Work out the finished part from the listing and answer in its coordinate system (mm). A direction names the side the tool comes from. Give positions to 0.01 mm unless a question says otherwise; leave off trailing zeros. Order: outer loops, then holes, each group sorted by start corner. A loop starts at its lowest first (then second) coordinate and runs counter-clockwise, first axis right, second up. Notation, with made-up numbers: (-36.75, 73) - (19.25, 73) arc R6 ccw to (19.25, 78) - close; hole circle Ø8 at (40.25, 50). An arc over 180 degrees is marked (long way). Write each question's results on one line, items separated by ' | '.
from build123d import *

# Parameters (mm, degrees)
SKETCH1_R           = 5
SKETCH1_R_2         = 2.5
BOSS_EXTRUDE2_DEPTH = 15
SKETCH2_W           = 6
SKETCH2_H           = 38.915837439
CUT_EXTRUDE1_DEPTH  = 11
CUT_EXTRUDE2_START  = -4.5
SKETCH3_R           = 4.6
SKETCH3_R_2         = 2.5
CUT_EXTRUDE2_DEPTH  = 6
CUT_EXTRUDE3_START  = -10.5
SKETCH4_R           = 4.6
SKETCH4_R_2         = 2.5
CUT_EXTRUDE3_DEPTH  = 6
BOSS_EXTRUDE3_DEPTH = 21
CUT_EXTRUDE4_DEPTH  = 67.015153021
BOSS_EXTRUDE4_START = -15.5
SKETCH8_R           = 6
BOSS_EXTRUDE4_DEPTH = 5.5


with BuildPart() as part:
    # Sketch1 → Boss-Extrude2 (new body)
    with BuildSketch(Plane(origin=(0, 0, 0), x_dir=(0, 0, -1), z_dir=(1, 0, 0))):
        with BuildLine():
            Line((0, -7), (4.514898748, -15.922762425))
            ThreePointArc((4.514898748, -15.922762425), (1.88507796, -23.910457261), (9.571950369, -20.5))
            Line((9.571950369, -20.5), (30.826440892, -20.5))
            ThreePointArc((30.826440892, -20.5), (36.979627599, -21.988417026), (38.792064121, -15.922762425))
            Line((38.792064121, -15.922762425), (38.792064121, 29.077237575))
            Line((38.792064121, 29.077237575), (17.792064121, 29.077237575))
            Line((17.792064121, 29.077237575), (17.792064121, 7))
            Line((17.792064121, 7), (0, 7))
            ThreePointArc((0, 7), (-7, 0), (0, -7))
        make_face()
        Circle(SKETCH1_R, mode=Mode.SUBTRACT)
        with Locations((4.971950369, -20.5)):
            Circle(SKETCH1_R_2, mode=Mode.SUBTRACT)
        with Locations((34.687787808, -18)):
            Circle(SKETCH1_R_2, mode=Mode.SUBTRACT)
    extrude(amount=BOSS_EXTRUDE2_DEPTH)

    # Sketch2 → Cut-Extrude1 (cut)
    with BuildSketch(Plane.XZ.offset(20.5)):
        with Locations((7.5, -19.829869089)):
            Rectangle(SKETCH2_W, SKETCH2_H)
    extrude(amount=-CUT_EXTRUDE1_DEPTH, mode=Mode.SUBTRACT)

    # Sketch3 → Cut-Extrude2 (cut)
    with BuildSketch(Plane.ZY.offset(CUT_EXTRUDE2_START)):
        with Locations((-4.971950369, -20.5)):
            Circle(SKETCH3_R)
        with Locations(Location((-4.971950369, -20.5, 0), (0, 0, 180))):
            Circle(SKETCH3_R_2, mode=Mode.SUBTRACT)
    extrude(amount=-CUT_EXTRUDE2_DEPTH, mode=Mode.SUBTRACT)

    # Sketch4 → Cut-Extrude3 (cut)
    with BuildSketch(Plane(origin=(15, 0, 0), x_dir=(0, 0, -1), z_dir=(1, 0, 0)).offset(CUT_EXTRUDE3_START)):
        with Locations((34.687787808, -18)):
            Circle(SKETCH4_R)
        with Locations((34.687787808, -18)):
            Circle(SKETCH4_R_2, mode=Mode.SUBTRACT)
    extrude(amount=CUT_EXTRUDE3_DEPTH, mode=Mode.SUBTRACT)

    # Sketch6 → Boss-Extrude3 (add)
    with BuildSketch(Plane(origin=(0, 0, -38.792064121), x_dir=(-1, 0, 0), z_dir=(0, 0, -1))):
        with BuildLine():
            ThreePointArc((0, 29.077237575), (-7.5, 44.40818947), (-15, 29.077237575))
            Line((-15, 29.077237575), (-8.914213562, 29.077237575))
            ThreePointArc((-8.914213562, 29.077237575), (-11.20909144, 39.624399885), (-1.5, 34.90818947))
            ThreePointArc((-1.5, 34.90818947), (-2.783789584, 31.199098029), (-6.085786438, 29.077237575))
            Line((-6.085786438, 29.077237575), (0, 29.077237575))
        make_face()
    extrude(amount=-BOSS_EXTRUDE3_DEPTH)

    # Sketch7 → Cut-Extrude4 (cut, through all)
    with BuildSketch(Plane(origin=(0, 0, -38.792064121), x_dir=(-1, 0, 0), z_dir=(0, 0, -1))):
        with BuildLine():
            Line((-8.914213562, 29.077237575), (-6.085786438, 29.077237575))
            ThreePointArc((-6.085786438, 29.077237575), (-7.5, 28.90818947), (-8.914213562, 29.077237575))
        make_face()
    extrude(amount=-CUT_EXTRUDE4_DEPTH, mode=Mode.SUBTRACT)

    # Sketch8 → Boss-Extrude4 (add)
    with BuildSketch(Plane(origin=(0, 0, -38.792064121), x_dir=(-1, 0, 0), z_dir=(0, 0, -1)).offset(BOSS_EXTRUDE4_START)):
        with Locations((-7.5, 34.90818947)):
            Circle(SKETCH8_R)
    extrude(amount=-BOSS_EXTRUDE4_DEPTH)


solid = part.part
1. A cutting plane is placed at A-A, the plane y = 0. Write down the section's boundary in (x, z).
Answer list:
outline: (0, -38.79) - (15, -38.79) - (15, -5) - (0, -5) - close; (0, 5) - (15, 5) - (15, 7) - (0, 7) - close
2. A cutting plane is placed at C-C, the plane z = -27. Write down the section's boundary in (x, y), then the cut area to 3 significant figures.
Answer list:
outline: (0, -20.5) - (4.5, -20.5) - (4.5, -9.5) - (10.5, -9.5) - (10.5, -20.5) - (15, -20.5) - (15, 29.08) arc R9.5 ccw (long way) to (0, 29.08) - close; hole circle Ø12 at (7.5, 34.91) | area: 810 mm^2
3. Given P1, Ø4, axis at x = 1, z = -6.5, coming from the +Y side; P2, Ø2, axis at x = 0, z = -34.5, coming from the +Y side; P3, Ø5, axis at y = 22, z = -27, coming from the -X side; P4, Ø6, axis at y = 0, z = 0, coming from the +X side, each flat-ended and moving along its own axis, determine where each tip first touches the part or whether it passes through.
Answer list:
P1: y = 7 | P2: y = 41.84 | P3: x = 0 | P4: through
4. A cutting plane is placed at B-B, the plane z = -36. Write down the section's boundary in (x, y), then the cut area to 3 significant figures.
Answer list:
outline: (0, -22.41) - (4.5, -22.41) - (4.5, -20.13) - (0, -20.13) - close; (0, -15.87) - (4.5, -15.87) - (4.5, -9.5) - (10.5, -9.5) - (10.5, -15.87) - (15, -15.87) - (15, 29.08) arc R9.5 ccw (long way) to (0, 29.08) - close; (10.5, -22.41) - (15, -22.41) - (15, -20.13) - (10.5, -20.13) - close; hole circle Ø12 at (7.5, 34.91) | area: 789 mm^2
5. A tool of negligible diameter and unlimited length cuts with its end or side. For faces 1 (the face through (7.4, -8.42, -0.72)), 2 (the face through (7, -9.5, -20)), 3 (the face through (13, -20.5, -20)), from which of +Z, -Z, +X, -X, +Y, -Y can it reach the whole face along a straight path? Write none if from no direction.
Answer list:
face 1: +Z, +X, -X | face 2: +Z, -Z, -Y | face 3: +X, -X, -Y
6. Determine the mould class of faces 4 (the face through (0, 2, -21)), 5 (the face through (4.5, -16, -20)), 6 (the face through (7, 0, 7)) for opening direction X: +X half, -X half, draft (parallel to the pull), parting line (faces both ways), or undercut.
Answer list:
face 4: -X half | face 5: undercut | face 6: draft
7. Straight lines are drawn through the part: line 1 (X direction, y = -14.5, z = -32.5); line 2 (Y direction, x = 6, z = 0); line 3 (Y direction, x = 7.25, z = -14). For each, find the intervals that lie inside material, in ascending order. Write a range as [from, to].
Answer list:
line 1: [0, 4.5], [10.5, 15] | line 2: [-7, -5], [5, 7] | line 3: [-9.5, 7]
8. A cutting plane is placed at D-D, the plane z = 1. Write down the section's boundary in (x, y), then the cut area to 3 significant figures.
Answer list:
outline: (0, -6.93) - (15, -6.93) - (15, -4.9) - (0, -4.9) - close; (0, 4.9) - (15, 4.9) - (15, 6.93) - (0, 6.93) - close | area: 60.9 mm^2
